The listing builds one solid part. Answer for the finished solid, in the listing's coordinates (mm). Give positions to 0.01 mm unless a question says otherwise; leave off trailing zeros. Write each loop counter-clockwise with the first axis right and the second up, starting at its lowest first coordinate (ties: lowest second). Pieces come first, ordered by that corner, then holes. Notation, with made-up numbers: M -17,50.25 L 2,50.25 A18 ccw 2,83.25 Z; hole C 75.25,47 d8. An arc over 180 degrees is marked long. Answer as a JSON object with one key per item and string values.
Autodesk Inventor part; units mm, degrees
ref_plane "YZ Plane" through (0, 0, 0) normal (1, 0, 0) x (0, 1, 0)
ref_plane "XZ Plane" through (0, 0, 0) normal (0, 1, 0) x (-1, 0, 0)
ref_plane "XY Plane" through (0, 0, 0) normal (0, 0, 1) x (1, 0, 0)
sketch "Sketch1" plane through (0, 0, 0) normal (0, 0, 1) x (1, 0, 0)
  circle A0 centre (-56.5936, 0) radius 1.5
  line L0 (-52.5936, 4) -> (-60.5936, 4)
  line L1 (-60.5936, 4) -> (-60.5936, -4)
  line L2 (-60.5936, -4) -> (-52.5936, -4)
  line L3 (-52.5936, -4) -> (-52.5936, 4)
  circle A1 centre (0, 0) radius 1.5
  line L4 (-4, 4) -> (-4, -4)
  line L5 (-4, -4) -> (4, -4)
  line L6 (4, -4) -> (4, 4)
  line L7 (4, 4) -> (-4, 4)
  line L8 (-60.5936, 4) -> (4, 4)
  line L9 (4, 4) -> (4, -4)
  line L10 (4, -4) -> (-60.5936, -4)
  line L11 (-60.5936, -4) -> (-60.5936, 4)
  point P0 (0, 0)
extrude "Extrusion1" add sketch "Sketch1" along normal blind 5
sketch "Sketch2" plane through (0, 0, 0) normal (0, 0, -1) x (-1, 0, 0)
  point P0 (0, 0)
sketch "Sketch3" plane through (0, 0, 0) normal (0, 0, -1) x (-1, 0, 0)
  line L0 (60.5936, 4) -> (60.5936, -4)
  line L1 (-4, 4) -> (60.5936, 4)
  line L2 (-4, -4) -> (-4, 4)
  line L3 (60.5936, -4) -> (-4, -4)
  circle A0 centre (0, 0) radius 1.5
  circle A1 centre (56.5936, 0) radius 1.5
  circle A2 centre (28.2966, 0) radius 1.95
  point P0 (0, 0)
  point P1 (60.5936, 0)
  dimension "d2" = 3.9
  dimension "d4" = 32.297
extrude "Extrusion2" cut sketch "Sketch3" against normal blind 1.8 contours A2
sketch "Sketch4" plane through (-28.2966, 0, 1.8) normal (0, 0, -1) x (-1, 0, 0)
  circle A0 centre (0, 0) radius 1
  point P0 (-28.2966, 0)
  dimension "d7" = 2
extrude "Extrusion3" cut sketch "Sketch4" against normal through all
properties part number "vertical_axis_hal_holder"
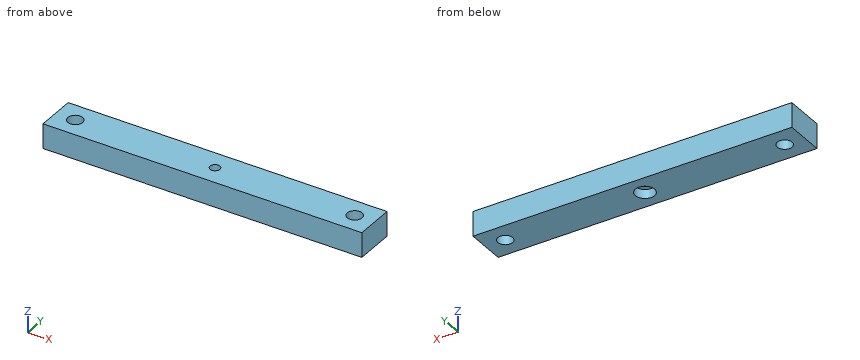
1. A cutting plane is placed at B-B, the plane y = 0. Give the vertices of the cut face in (x, z), plus the area to 3 significant figures.
Verdict:
{"outline": "M -60.59,0 L -58.09,0 L -58.09,5 L -60.59,5 Z; M -55.09,0 L -30.25,0 L -30.25,1.8 L -29.3,1.8 L -29.3,5 L -55.09,5 Z; M -27.3,1.8 L -26.35,1.8 L -26.35,0 L -1.5,0 L -1.5,5 L -27.3,5 Z; M 1.5,0 L 4,0 L 4,5 L 1.5,5 Z", "area": "280 mm2"}
2. A cutting plane is placed at C-C, the plane z = 0.75. Give the vertices of the cut face in (x, y).
Verdict:
{"outline": "M -60.59,-4 L 4,-4 L 4,4 L -60.59,4 Z; hole C -56.59,0 d3; hole C -28.3,0 d3.9; hole C 0,0 d3"}
3. A cutting plane is placed at A-A, the plane x = 0. Give the vertices of the cut face in (y, z).
Verdict:
{"outline": "M -4,0 L -1.5,0 L -1.5,5 L -4,5 Z; M 1.5,0 L 4,0 L 4,5 L 1.5,5 Z"}
4. A flat-ended cylindrical pin translates along its axis: pin 1 (3 mm diameter, centred on x = -28.5, y = 0, fed in from -Z). Find the tip coordinate at first contact, or state that the pin passes through.
Verdict:
{"pin 1": "stops at z = 1.8"}
5. A cutting plane is placed at D-D, the plane z = 3.9. Give the vertices of the cut face in (x, y).
Verdict:
{"outline": "M -60.59,-4 L 4,-4 L 4,4 L -60.59,4 Z; hole C -56.59,0 d3; hole C -28.3,0 d2; hole C 0,0 d3"}
6. Consider line 1 along Y through (x, z) = (0, 3.8); line 2 along X through (y, z) = (0.75, 3.6); line 3 along Y through (x, z) = (-28, 4.8) (3 decimals). Determine where each line is inside the solid, lowest interval first.
Verdict:
{"line 1": "y = -4 to -1.5, 1.5 to 4", "line 2": "x = -60.59 to -57.89, -55.29 to -28.96, -27.64 to -1.3, 1.3 to 4", "line 3": "y = -4 to -0.955, 0.955 to 4"}
